Here's how the part is built. I have some questions about the finished solid (model axes, mm). A direction names the side the tool comes from. Give positions to 0.01 mm unless a question says otherwise; leave off trailing zeros. Loops run counter-clockwise (first coordinate to the right, second up) from the corner with the lowest first, then second, coordinate; pieces in that order, holes last. Notation, with made-up numbers: (84.25, 54) - (124.25, 54) arc R19 ccw to (124.25, 61) - close; hole circle Ø8 at (2, 57). An arc over 180 degrees is marked (long way). Use one line per item in the form item = value.
from build123d import *

# Parameters (mm, degrees)
F1_DEPTH = 304.8
F3_DEPTH = 50.8
F4_R     = 5.07999


# Not quite as in the source:
# - a fillet or chamfer is up to 0.001 mm smaller than in the source, because OpenCascade refuses the exact size


with BuildPart() as f1:
    # F0 (on Front) → F1 (new body)
    with BuildSketch(Plane.XZ):
        Polygon((50.8, 0), (0, 0), (0, -22.86), (7.62, -22.86), (7.62, -27.94), (17.78, -27.94), (17.78, -35.56), (20.32, -35.56), (20.32, -30.48), (35.56, -30.48), (35.56, -35.56), (38.1, -35.56), (38.1, -12.7), (50.8, -12.7), align=None)
    extrude(amount=F1_DEPTH)

    # F2 (on face) → F3 (cut)
    with BuildSketch(Plane(origin=(0, 0, 0), x_dir=(0, -1, 0), z_dir=(-1, 0, 0))):
        Polygon((35.56, -35.56), (0, 0), (0, -35.56), align=None)
        Polygon((304.8, -35.56), (304.8, 0), (269.24, -35.56), align=None)
    extrude(amount=-F3_DEPTH, mode=Mode.SUBTRACT)

    # F4 (radius 5.08 in the source; OpenCascade refuses exactly that, so slightly less here)
    f4_edges = [f1.edges().sort_by_distance(p)[0] for p in [
        (7.62, -152.4, -27.94),
    ]]
    fillet(f4_edges, radius=F4_R)


solid = f1.part
(1) If I drill on probe 1 along X at (y, z) = (-181, -33.5); probe 2 along Z at (x, y) = (34, -183); probe 3 along Z at (x, y) = (39, -85.5), over which ranges is the centre line in solid material (lowest first)?
Geometry says:
probe_1 = 17.78 to 20.32, 35.56 to 38.1
probe_2 = -30.48 to 0
probe_3 = -12.7 to 0
(2) If we section it at B-B (x = 25): List the corners of the cut face in (y, z) for me.
Geometry says:
outline = (-304.8, 0) - (-274.32, -30.48) - (-30.48, -30.48) - (0, 0) - close
(3) If we section it at C-C (z = -3): List the corners of the cut face in (x, y) for me, plus the area to 3 significant figures.
Geometry says:
outline = (0, -301.8) - (50.8, -301.8) - (50.8, -3) - (0, -3) - close
area = 15,200 mm²
(4) If we section it at D-D (y = -285.5): List the corners of the cut face in (x, z) for me.
Geometry says:
outline = (0, -19.3) - (38.1, -19.3) - (38.1, -12.7) - (50.8, -12.7) - (50.8, 0) - (0, 0) - close
(5) For faces 5 (the flat face through (44, -150, -12.7)), 6 (the flat face through (50.8, -150, -6)), 7 (the flat face through (35.56, -151, -33)), 8 (the flat face through (15, -151, -27.94)), which set-ups out of +Z, -Z, +X, -X, +Y, -Y let a thin tool reach every point of the face, with its end or its side?
Geometry says:
face_5 = -Z, +X, +Y, -Y
face_6 = +Z, -Z, +X, +Y, -Y
face_7 = -Z, +Y, -Y
face_8 = -Z, -X, +Y, -Y
(6) Thinking about a two-plate mould opening in X: for faces 1 (the flat face through (26, -150, 0)), 2 (the flat face through (0, -150, -11)), 3 (the flat face through (28, -151, -30.48)), 4 (the flat face through (20.32, -151, -33)), which applies, pulls with the +X half, pulls with the -X half, needs draft (parallel to the pull), parting line crosses it, or undercut?
Geometry says:
face_1 = needs draft
face_2 = pulls with the -X half
face_3 = undercut
face_4 = undercut
(7) For P1, Ø1.5, axis at x = 27.5, z = -26, coming from the -Y side; P2, Ø1.5, axis at x = 33, z = -15.5, coming from the -Y side; P3, Ø1.5, axis at y = -110.5, z = -32, coming from the -X side, each with a flat end and sliding along its axis, tell me the tip position at first contact or that it passes through.
Geometry says:
P1 = -279.55
P2 = -290.05
P3 = 17.78
